Read the model definition and answer for the solid it produces. Units are mm, in the model's axes. Face numbers are marked on the shaded views. A direction names the side the tool comes from. Give positions to 0.01 mm unless a question says otherwise; leave off trailing zeros. Write each loop counter-clockwise with the first axis right and the second up, starting at its lowest first coordinate (ties: lowest second). Pieces come first, ordered by that corner, then holes. Notation, with made-up numbers: M -32.5,-31 L 19.5,-31 A25 cw 19.5,3 Z; hole C 21,14.25 d2. An arc over 180 degrees is marked long. Write each question's results on one line, items separated by ' | '. Start each with the question number.
```python
from build123d import *

# Parameters (mm, degrees)
SKETCH2_R               = 15
BOSS_EXTRUDE1_DEPTH     = 25
SKETCH7_W               = 5
SKETCH7_H               = 30
BOSS_EXTRUDE2_DEPTH     = 4
BOSS_EXTRUDE3_DEPTH     = 5
CUT_EXTRUDE3_DEPTH      = 35.003676272
CUT_EXTRUDE3_DEPTH_BACK = 35.003676272
SKETCH9_R               = 2.5


with BuildPart() as part:
    # Sketch2 → Boss-Extrude1 (new body)
    with BuildSketch(Plane(origin=(0, 0, 0), x_dir=(0, 0, -1), z_dir=(1, 0, 0))):
        Circle(SKETCH2_R)
    extrude(amount=-BOSS_EXTRUDE1_DEPTH)

    # Sketch7 → Boss-Extrude2 (add)
    with BuildSketch(Plane(origin=(0, 0, 0), x_dir=(0, 0, -1), z_dir=(1, 0, 0))):
        Rectangle(SKETCH7_W, SKETCH7_H)
    extrude(amount=BOSS_EXTRUDE2_DEPTH)

    # Sketch8 → Boss-Extrude3 (add)
    with BuildSketch(Plane.XY.offset(2.5)):
        with BuildLine():
            Line((4, 15), (4, -15))
            ThreePointArc((4, -15), (19, 0), (4, 15))
        make_face()
    extrude(amount=-BOSS_EXTRUDE3_DEPTH)

    # Sketch9 → Cut-Extrude3 (cut, two sides: drawn at the far end of the back side and taken through both)
    with BuildSketch(Plane.XY.offset(2.5).offset(-CUT_EXTRUDE3_DEPTH_BACK)):
        with Locations(Location((14, 0, 0), (0, 0, 270))):
            Circle(SKETCH9_R)
    extrude(amount=CUT_EXTRUDE3_DEPTH + CUT_EXTRUDE3_DEPTH_BACK, mode=Mode.SUBTRACT)

    # Sketch10 → Revolve1 (revolve)
    with BuildSketch(Plane.ZY.offset(25)):
        with BuildLine():
            Line((0, 15), (0, -15))
            ThreePointArc((0, -15), (15, 0), (0, 15))
        make_face()
    revolve(axis=Axis((-25, 15, 0), (0, -1, 0)))


solid = part.part
```
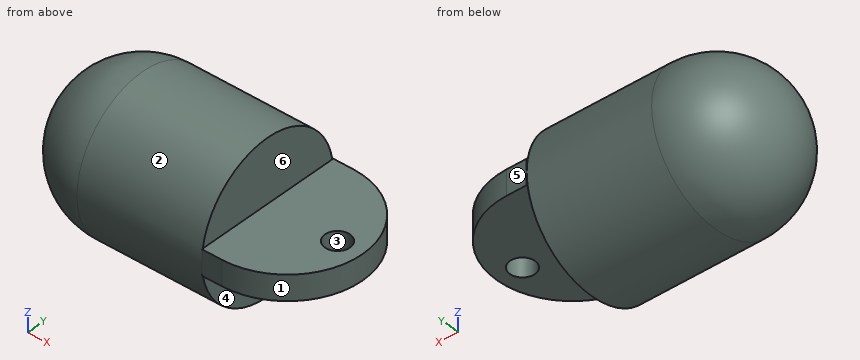
Item 1: Section B-B, the plane x = 15 is taken. Determine the outline of the cut face in (y, z).
Item 2: Determine the mould class of the marked faces 1, 2 and 3 for opening direction X: +X half, -X half, draft (parallel to the pull), parting line (faces both ways), or undercut.
Item 3: For the marked faces 4, 5 and 6, determine the directions among +Z, -Z, +X, -X, +Y, -Y from which every point of the face is accessible in a straight line to the end or side of a thin tool.
Item 4: Straight lines are drawn through the part: line 1 (X direction, y = 0, z = -0.2); line 2 (Z direction, x = 3.5, y = 8.75); line 3 (X direction, y = -1.25, z = -1.5). For each, find the intervals that lie inside material, in ascending order.
Item 5: Section A-A, the plane y = 0 is taken. Determine the outline of the cut face in (x, z).
Item 6: Section D-D, the plane z = -8.75 is taken. Determine the outline of the cut face in (x, y), then the cut area to 3 significant figures.
Item 7: Section C-C, the plane y = 9 is taken. Determine the outline of the cut face in (x, z), then the cut area to 3 significant figures.
Item 8: Given P1, Ø1, axis at x = 12, z = -1, coming from the -Y side; P2, Ø1.5, axis at y = 2.5, z = -10, coming from the +X side; P3, Ø8, axis at x = 14, y = 0, coming from the -Z side, each flat-ended and moving along its own axis, determine where each tip first touches the part or whether it passes through.
Worked out:
1) outline: M -10.2,-2.5 L -2.29,-2.5 L -2.29,2.5 L -10.2,2.5 Z; M 2.29,-2.5 L 10.2,-2.5 L 10.2,2.5 L 2.29,2.5 Z
2) face 1: +X half | face 2: draft | face 3: undercut
3) face 4: -Z, +X, +Y, -Y | face 5: +Z, -Z, +X, -X, +Y | face 6: +Z, +X, +Y, -Y
4) line 1: x = -40 to 11.5, 16.5 to 19 | line 2: z = -2.5 to 2.5 | line 3: x = -39.87 to 11.83, 16.17 to 18.95
5) outline: M -25,-15 L 0,-15 L 0,-2.5 L 11.5,-2.5 L 11.5,2.5 L 0,2.5 L 0,15 L -25,15 A15 ccw Z; M 16.5,-2.5 L 19,-2.5 L 19,2.5 L 16.5,2.5 Z
6) outline: M -25,-12.18 L 0,-12.18 L 0,12.18 L -25,12.18 A12.18 ccw Z | area: 842 mm²
7) outline: M -25,-12 L 0,-12 L 0,-2.5 L 16,-2.5 L 16,2.5 L 0,2.5 L 0,12 L -25,12 A12 ccw Z | area: 906 mm²
8) P1: stops at y = -12.99 | P2: stops at x = 0 | P3: stops at z = -2.5
